Source: CAD feature listing. Evaluate the final solid. Frame: model axes, mm. Face numbers are marked on the shaded views. A direction names the side the tool comes from. Coordinates: 2 decimals unless noted, no trailing zeros. Write each loop counter-clockwise with the first axis right and the second up, starting at its lowest first coordinate (ties: lowest second). Pieces come first, ordered by that corner, then holes. Notation, with made-up numbers: M -38,-27.75 L -15,-27.75 A13 cw -15,-5.75 Z; hole C 14.5,71 d6. An arc over 180 degrees is marked long. Write item = value, one per line. Start each with the question number.
1. Line query: line 1 along Y through (x, z) = (-2.1, 0); line 2 along Y through (x, z) = (-0.3, -0.6); line 3 along Z through (x, y) = (-1.9, -3.25). Output: solid intervals per line, ascending.
2. Section query D-D (x = 2). Output: boundary loops of the cut face in (y, z), then the cut area to 3 significant figures.
3. Pin query (flat end, axial travel): pin 1 Ø0.7 at (x, y) = (0.5, -3) entering from +Z; pin 2 Ø1 at (x, y) = (1, 10.5) entering from +Z; pin 3 Ø2 at (x, y) = (-2, 8) entering from +Z. Return the tip coordinate at first contact, or that it passes through.
4. Access query for the marked faces 4, 5 and 6. Directions: +Z, -Z, +X, -X, +Y, -Y. A direction counts if a zero-diameter tool reaches every point of the face in a straight line with its end or side. Return the directions, or none.
5. Section query B-B (z = -1.15). Output: boundary loops of the cut face in (x, y), then the cut area to 3 significant figures.
6. Section query C-C (y = 1.75). Output: boundary loops of the cut face in (x, z).
7. Section query A-A (x = 0). Output: boundary loops of the cut face in (y, z), then the cut area to 3 significant figures.
8. Pull-direction query (X, two-part tool) for the marked faces 1, 2 and 3; classes: pulls with the +X half, pulls with the -X half, needs draft (parallel to the pull), parting line crosses it, or undercut.
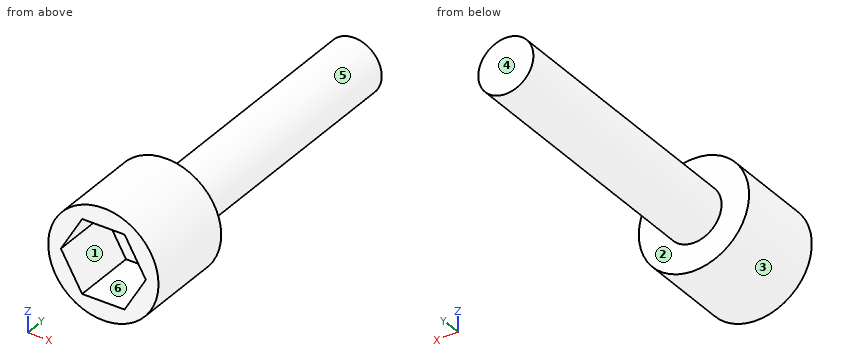
```python
from build123d import *

# Parameters (mm, degrees)
F0_R     = 3
F1_DEPTH = 5
F3_DEPTH = 3.5
F4_R     = 1.5
F5_DEPTH = 15


with BuildPart() as f1:
    # F0 (on Front) → F1 (new body)
    with BuildSketch(Plane.XZ):
        Circle(F0_R)
    extrude(amount=F1_DEPTH)

    # F2 (on face) → F3 (cut)
    with BuildSketch(Plane.XZ.offset(5)):
        Polygon((1.154701, 2), (-1.154701, 2), (-2.309401, 0), (-1.154701, -2), (1.154701, -2), (2.309401, 0), align=None)
    extrude(amount=-F3_DEPTH, mode=Mode.SUBTRACT)

    # F4 (on face) → F5 (join)
    with BuildSketch(Plane(origin=(0, 0, 0), x_dir=(-1, 0, 0), z_dir=(0, 1, 0))):
        Circle(F4_R)
    extrude(amount=F5_DEPTH)


solid = f1.part
```
Results are:
q1.line_1 = -1.5 to 0
q1.line_2 = -1.5 to 15
q1.line_3 = -2.32 to -0.71, 0.71 to 2.32
q2.outline = M -5,-2.24 L 0,-2.24 L 0,2.24 L -5,2.24 L -5,0.54 L -1.5,0.54 L -1.5,-0.54 L -5,-0.54 Z
q2.area = 18.6 mm^2
q3.pin_1 = 3
q3.pin_2 = 1.41
q3.pin_3 = 1.12
q4.face_4 = +Z, -Z, +X, -X, +Y
q4.face_5 = +Y
q4.face_6 = -Y
q5.outline = M -2.77,-5 L -1.65,-5 L -1.65,-1.5 L 1.65,-1.5 L 1.65,-5 L 2.77,-5 L 2.77,0 L 0.96,0 L 0.96,15 L -0.96,15 L -0.96,0 L -2.77,0 Z
q5.area = 45.1 mm^2
q6.outline = C 0,0 d3
q7.outline = M -5,-3 L 0,-3 L 0,-1.5 L 15,-1.5 L 15,1.5 L 0,1.5 L 0,3 L -5,3 L -5,2 L -1.5,2 L -1.5,-2 L -5,-2 Z
q7.area = 61.0 mm^2
q8.face_1 = undercut
q8.face_2 = needs draft
q8.face_3 = parting line crosses it
